Answer from the drawing. Dimensions are ordinates in mm from the lowest x, y and z of the part. A direction names the side the tool comes from. Give positions to 0.01 mm unless a question says otherwise; leave off trailing zeros. Order: outer loops, then holes, each group sorted by start corner. A loop starts at its lowest first (then second) coordinate and runs counter-clockwise, first axis right, second up. Notation, with made-up numbers: (2, 38.25) - (29, 38.25) arc R23 cw to (29, 76.25) - close; hole circle Ø5 at (52.5, -4). An arc over 180 degrees is marked (long way). Use a Markdown table: item, result. Add a question column.
1) The mould has two halves that part along Y. Classify the marked faces 3, 4 and 5: released by +Y, released by -Y, zero draft, split by the parting line, or undercut.
2) Straight lines are drawn through the part: line 1 (X direction, y = 23, z = 47); line 2 (Y direction, x = 6, z = 38) (1 decimal); line 3 (Z direction, x = 183, y = 57.15) (1 decimal). For each, find the intervals that lie inside material, in ascending order.
3) For the marked faces 1 and 2, determine the directions among +Z, -Z, +X, -X, +Y, -Y from which every point of the face is accessible in a straight line to the end or side of a thin tool.
4) A flat-ended cylindrical pin translates along its axis: pin 1 (4 mm diameter, centred on x = 128.5, y = 102.5, fed in from +Z). Find the tip coordinate at first contact, or state that the pin passes through.
5) Find section A-A, the plane y = 57.15. Determine the outline of the cut face in (x, z) (1 decimal), plus the area to 3 significant figures.
6) Find section D-D, the plane y = 31. Determine the outline of the cut face in (x, z).
7) Find section B-B, the plane z = 19.5. Determine the outline of the cut face in (x, y).
8) Find section C-C, the plane x = 44.5. Determine the outline of the cut face in (y, z).
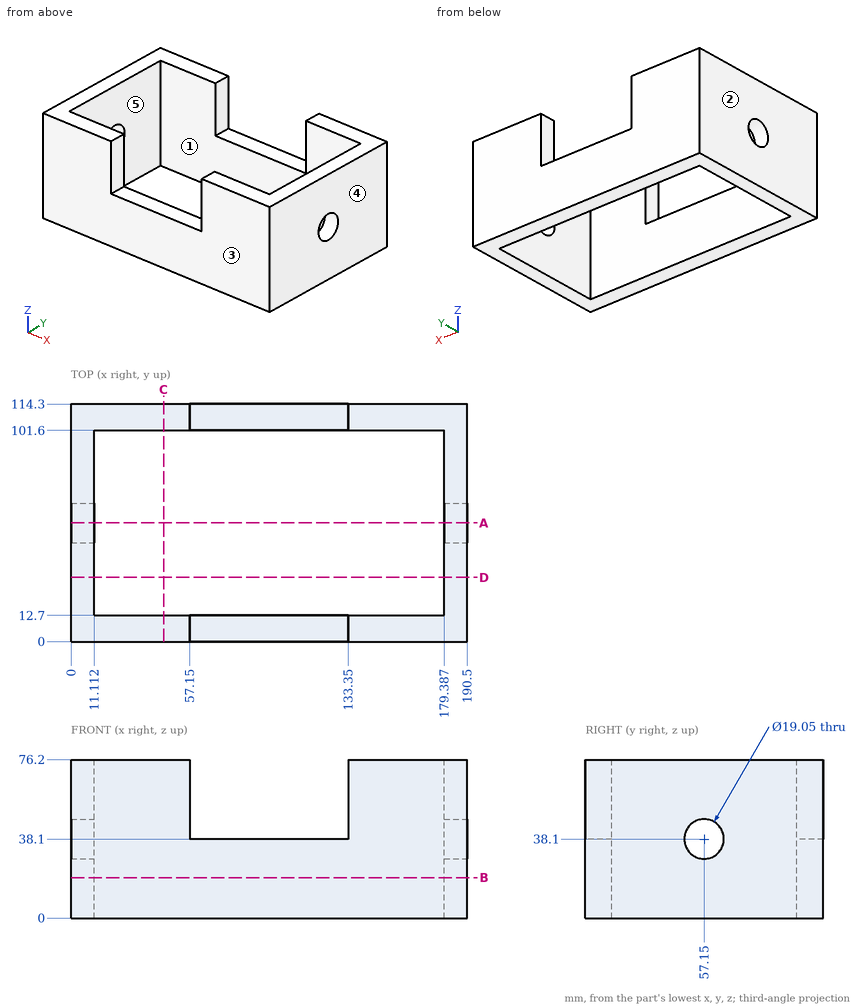
The answers:
| question | item | result |
|---|---|---|
| 1 | face 3 | released by -Y |
| 1 | face 4 | zero draft |
| 1 | face 5 | undercut |
| 2 | line 1 | 0 to 11.11, 179.39 to 190.5 |
| 2 | line 2 | 0 to 47.6, 66.7 to 114.3 |
| 2 | line 3 | 0 to 28.6, 47.6 to 76.2 |
| 3 | face 1 | +Z, -Z |
| 3 | face 2 | +Z, -Z, -X, +Y, -Y |
| 4 | pin 1 | z = 38.1 |
| 5 | outline | (0, 0) - (11.1, 0) - (11.1, 28.6) - (0, 28.6) - close; (0, 47.6) - (11.1, 47.6) - (11.1, 76.2) - (0, 76.2) - close; (179.4, 0) - (190.5, 0) - (190.5, 28.6) - (179.4, 28.6) - close; (179.4, 47.6) - (190.5, 47.6) - (190.5, 76.2) - (179.4, 76.2) - close |
| 5 | area | 1,270 mm2 |
| 6 | outline | (0, 0) - (11.11, 0) - (11.11, 76.2) - (0, 76.2) - close; (179.39, 0) - (190.5, 0) - (190.5, 76.2) - (179.39, 76.2) - close |
| 7 | outline | (0, 0) - (190.5, 0) - (190.5, 114.3) - (0, 114.3) - close; hole (11.11, 12.7) - (179.39, 12.7) - (179.39, 101.6) - (11.11, 101.6) - close |
| 8 | outline | (0, 0) - (12.7, 0) - (12.7, 76.2) - (0, 76.2) - close; (101.6, 0) - (114.3, 0) - (114.3, 76.2) - (101.6, 76.2) - close |
